from build123d import *

# Parameters (mm, degrees)
SKETCH1_R           = 16
BOSS_EXTRUDE1_DEPTH = 22.5
BOSS_EXTRUDE2_DEPTH = 3
SKETCH3_R           = 1.5
BOSS_EXTRUDE3_DEPTH = 10
SKETCH4_R           = 14
CUT_EXTRUDE1_DEPTH  = 23.5
SKETCH5_R           = 1.5
CUT_EXTRUDE2_DEPTH  = 51.00499975
SKETCH7_R           = 5
BOSS_EXTRUDE4_DEPTH = 3
FILLET1_R           = 2


with BuildPart() as part:
    # Sketch1 → Boss-Extrude1 (new body)
    with BuildSketch(Plane(origin=(0, 0, 0), x_dir=(1, 0, 0), z_dir=(0, 1, 0))):
        with Locations(Location((0, 0, 0), (0, 0, 90))):
            Circle(SKETCH1_R)
    extrude(amount=BOSS_EXTRUDE1_DEPTH)

    # Sketch2 → Boss-Extrude2 (add)
    with BuildSketch(Plane(origin=(0, 22.5, 0), x_dir=(1, 0, 0), z_dir=(0, 1, 0))):
        with BuildLine():
            Line((-16, -17.5), (-16, 17.5))
            ThreePointArc((-16, 17.5), (0, 33.5), (16, 17.5))
            Line((16, 17.5), (16, -17.5))
            ThreePointArc((16, -17.5), (0, -33.5), (-16, -17.5))
        make_face()
    extrude(amount=BOSS_EXTRUDE2_DEPTH)

    # Sketch3 → Boss-Extrude3 (add)
    with BuildSketch(Plane(origin=(0, 25.5, 0), x_dir=(1, 0, 0), z_dir=(0, 1, 0))):
        with Locations(Location((0, 25, 0), (0, 0, 270))):
            Circle(SKETCH3_R)
        with Locations(Location((0, -25, 0), (0, 0, 270))):
            Circle(SKETCH3_R)
    extrude(amount=BOSS_EXTRUDE3_DEPTH)

    # Sketch4 → Cut-Extrude1 (cut)
    with BuildSketch(Plane(origin=(0, 25.5, 0), x_dir=(1, 0, 0), z_dir=(0, 1, 0))):
        with Locations(Location((0, 0, 0), (0, 0, 270))):
            Circle(SKETCH4_R)
    extrude(amount=-CUT_EXTRUDE1_DEPTH, mode=Mode.SUBTRACT)

    # Sketch5 → Cut-Extrude2 (cut, through all)
    with BuildSketch(Plane(origin=(0, 2, 0), x_dir=(1, 0, 0), z_dir=(0, 1, 0))):
        with Locations(Location((8, 0, 0), (0, 0, 270))):
            Circle(SKETCH5_R)
        with Locations(Location((-8, 0, 0), (0, 0, 270))):
            Circle(SKETCH5_R)
    extrude(amount=-CUT_EXTRUDE2_DEPTH, mode=Mode.SUBTRACT)

    # Sketch7 → Boss-Extrude4 (add)
    with BuildSketch(Plane(origin=(0, 35.5, 0), x_dir=(1, 0, 0), z_dir=(0, 1, 0))):
        with Locations(Location((0, 25, 0), (0, 0, 270))):
            Circle(SKETCH7_R)
        with Locations(Location((0, -25, 0), (0, 0, 270))):
            Circle(SKETCH7_R)
    extrude(amount=BOSS_EXTRUDE4_DEPTH)

    # Fillet1
    fillet1_edges = [part.edges().sort_by_distance(p)[0] for p in [
        (0, 25.5, -26.5),
        (0, 35.5, -26.5),
        (0, 25.5, 23.5),
        (0, 35.5, 23.5),
    ]]
    fillet(fillet1_edges, radius=FILLET1_R)


solid = part.part
For this review, take the finished solid that the model builds, in its own axes (mm). A direction names the side the tool comes from. Round coordinates to 2 decimals unless told otherwise and drop trailing zeros. Loops run counter-clockwise (first coordinate to the right, second up) from the corner with the lowest first, then second, coordinate; pieces in that order, holes last. Notation, with made-up numbers: (58.25, 78.25) - (67.25, 78.25) arc R18 cw to (67.25, 86.25) - close; hole circle Ø6 at (-2.5, 24). An arc over 180 degrees is marked (long way). Answer as CSV lines item,"result".
(1) Wall thickness on line 1 (X direction, y = 1.35, z = 0); line 2 (Y direction, x = 2.5, z = 16.5); line 3 (X direction, y = 6.5, z = -11): over which ranges is each line inside the solid? List them lowest first.
Checked values:
line 1,"x = -16 to -9.5, -6.5 to 6.5, 9.5 to 16"
line 2,"y = 22.5 to 25.5"
line 3,"x = -11.62 to -8.66, 8.66 to 11.62"
(2) Consider section B-B on x = 8. Give the boundary of the cut face in (y, z).
Checked values:
outline,"(0, -13.86) - (22.5, -13.86) - (22.5, -31.36) - (25.5, -31.36) - (25.5, -11.49) - (2, -11.49) - (2, -1.5) - (0, -1.5) - close; (0, 1.5) - (2, 1.5) - (2, 11.49) - (25.5, 11.49) - (25.5, 31.36) - (22.5, 31.36) - (22.5, 13.86) - (0, 13.86) - close"
(3) Tool access review of faces 4 (the face through (15.62, 11.09, 3.47)), 5 (the face through (0, 37, -30)), 6 (the face through (-3.3, 35.5, -22.8)), 7 (the face through (0, 0, 0)): name each direction out of +Z, -Z, +X, -X, +Y, -Y from which nothing blocks a thin tool from reaching the whole face with its end or side.
Checked values:
face 4,"-Y"
face 5,"+Y"
face 6,"none"
face 7,"+Z, -Z, +X, -X, -Y"
(4) Consider section A-A on y = 32.5. Give the boundary of the cut face in (x, z), then the cut area to 3 significant figures.
Checked values:
outline,"circle Ø3 at (0, -25); circle Ø3 at (0, 25)"
area,"14.1 mm2"
(5) Consider section C-C on z = -25. Give the boundary of the cut face in (x, y).
Checked values:
outline,"(-14.13, 22.5) - (14.13, 22.5) - (14.13, 25.5) - (3.5, 25.5) arc R2 cw to (1.5, 27.5) - (1.5, 33.5) arc R2 cw to (3.5, 35.5) - (5, 35.5) - (5, 38.5) - (-5, 38.5) - (-5, 35.5) - (-3.5, 35.5) arc R2 cw to (-1.5, 33.5) - (-1.5, 27.5) arc R2 cw to (-3.5, 25.5) - (-14.13, 25.5) - close"
(6) Consider section D-D on y = 12. Give the boundary of the cut face in (x, z), then the cut area to 3 significant figures.
Checked values:
outline,"circle Ø32 at (0, 0); hole circle Ø28 at (0, 0)"
area,"188 mm2"
(7) Insertion check: P1, Ø10, axis at x = -11, y = 20, coming from the +Z side; P2, Ø8, axis at x = -2, z = 25, coming from the -Y side; P3, Ø2, axis at x = 5, z = -12.5, coming from the +Y side; P4, Ø1.8, axis at x = -8, z = 0, coming from the -Y side. Each pin has a flat end and moves straight along its axis. Give the tip position at first contact, or say it passes through.
Checked values:
P1,"stops at z = 32.04"
P2,"stops at y = 22.5"
P3,"stops at y = 25.5"
P4,"passes through"
(8) Mouldability with a two-part tool opening along X and no side actions: class faces 1 (the face through (0.352, 23.979, 33.496)), 2 (the face through (-3.3, 35.5, 27.2)), 3 (the face through (6.536, 1.014, -0.325)) as +X half, -X half, draft (parallel to the pull), parting line (faces both ways), or undercut.
Checked values:
face 1,"parting line"
face 2,"draft"
face 3,"undercut"
